Work out the finished part from the listing and answer in its coordinate system (mm). A direction names the side the tool comes from. Round coordinates to 2 decimals unless told otherwise and drop trailing zeros. Write each loop counter-clockwise with the first axis right and the second up, starting at its lowest first coordinate (ties: lowest second). Pieces come first, ordered by that corner, then holes. Notation, with made-up numbers: (46.5, 79.25) - (85.5, 79.25) arc R33 ccw to (85.5, 109.25) - close; hole circle Ø9 at (28, -22). An arc over 180 degrees is marked (long way). Answer as a JSON object with one key per item and string values.
Autodesk Inventor part; units mm, degrees
ref_plane "Work Plane1" through (0, 18.542, 0) normal (0, 1, 0) x (1, 0, 0)
ref_plane "YZ Plane" through (0, 0, 0) normal (1, 0, 0) x (0, 1, 0)
ref_plane "XZ Plane" through (0, 0, 0) normal (0, 1, 0) x (-1, 0, 0)
sketch "Sketch1" plane through (0, 0, 0) normal (0, 1, 0) x (-1, 0, 0)
  line L0 (1.27, 0) -> (11.43, 0)
  line L1 (12.7, -1.27) -> (12.7, -21.59)
  line L2 (11.43, -22.86) -> (1.27, -22.86)
  line L3 (0, -21.59) -> (0, -1.27)
  arc A0 (12.7, -1.27) -> (11.43, 0) centre (11.43, -1.27) ccw
  arc A1 (1.27, 0) -> (0, -1.27) centre (1.27, -1.27) ccw
  arc A2 (0, -21.59) -> (1.27, -22.86) centre (1.27, -21.59) ccw
  arc A3 (11.43, -22.86) -> (12.7, -21.59) centre (11.43, -21.59) ccw
  point P0 (0, 0)
  point P1 (12.7, -22.86)
  point P2 (12.7, 0)
  point P3 (0, -22.86)
  dimension "d0" = 12.7
  dimension "d1" = 22.86
  dimension "d2" = 1.27
extrude "Extrusion1" add sketch "Sketch1" along normal blind 22.86
sketch "Sketch2" plane through (0, 22.86, 0) normal (0, 1, 0) x (1, 0, 0)
  line L0 (-12.7, 21.59) -> (-12.7, 1.27)
  line L1 (-11.43, 0) -> (-1.27, 0)
  line L2 (0, 1.27) -> (0, 21.59)
  circle A0 centre (-6.35, 6.35) radius 6.35
  point P0 (0, 0)
extrude "Extrusion2" add sketch "Sketch2" along normal blind 5.08
ref_plane "Work Plane1" through (0, 18.542, 0) normal (0, 1, 0) x (1, 0, 0)
sketch "Sketch5" plane through (0, 18.542, 0) normal (0, 1, 0) x (1, 0, 0)
  line L0 (-12.7, 27.432) -> (0, 27.432)
  line L1 (-12.7, 21.59) -> (-12.7, 1.27)
  line L2 (0, 1.27) -> (0, 21.59)
  circle A0 centre (-6.35, 24.13) radius 1.016
  line L3 (0, 11.43) -> (-12.7, 11.43) construction
  line L4 (-12.7, -4.572) -> (0, -4.572)
  circle A1 centre (-6.35, -1.27) radius 1.016
  line L5 (-12.7, -4.572) -> (-12.7, 27.432)
  line L6 (0, 27.432) -> (0, -4.572)
  point P0 (0, 0)
  dimension "d13" = 16.002
  dimension "d14" = 2.032
  dimension "d15" = 25.4
extrude "Extrusion4" add sketch "Sketch5" against normal blind 2.54
sketch "Sketch6" plane through (-11.43, 0, 0) normal (0, 0, 1) x (1, 0, 0)
  line L0 (3.429, 5.334) -> (6.731, 5.334)
  line L1 (6.731, 5.334) -> (6.731, 4.318)
  line L2 (6.731, 4.318) -> (3.429, 4.318)
  line L3 (3.429, 4.318) -> (3.429, 5.334)
  line L4 (0, 0) -> (10.16, 0)
  point P0 (11.43, 0)
  point P1 (5.08, 0)
  point P2 (5.08, 4.318)
  dimension "d18" = 3.302
  dimension "d19" = 1.016
  dimension "d20" = 4.318
extrude "Extrusion5" add sketch "Sketch6" along normal blind 2.54
sketch "Sketch7" plane through (-6.35, 27.94, -6.35) normal (0, 1, 0) x (1, 0, 0)
  circle A0 centre (0, 0) radius 2.5
  point P0 (6.35, -6.35)
  dimension "d23" = 5
extrude "Extrusion6" add sketch "Sketch7" along normal blind 4.064
properties part number "Servo_With_Attachment"
Item 1: Determine the mould class of faces 1 (the cylindrical face through (-8.334, 29.944, -7.871)), 2 (the flat face through (-6, 8, 0)), 3 (the flat face through (-3.6, 27.94, -6.4)) for opening direction Y: pulls with the +Y half, pulls with the -Y half, needs draft (parallel to the pull), parting line crosses it, or undercut.
Results found:
{"face 1": "needs draft", "face 2": "undercut", "face 3": "pulls with the +Y half"}
Item 2: For faces 4 (the flat face through (-6, 8, -22.86)), 5 (the cylindrical face through (-12.338, 20.671, -22.478)), 6 (the flat face through (-6, 5.334, 1)), 7 (the flat face through (-2, 22.86, -1)), 8 (the flat face through (-11.2, 22.86, -1.5)), determine the directions among +Z, -Z, +X, -X, +Y, -Y from which every point of the face is accessible in a straight line to the end or side of a thin tool.
Results found:
{"face 4": "-Z, +X, -X, -Y", "face 5": "-Z, -X, +Y", "face 6": "+Z, +X, -X", "face 7": "+Z, +X, +Y", "face 8": "+Z, -X, +Y"}
Item 3: A cutting plane is placed at A-A (z = 1.27). Write down the section's boundary in (x, y), and give its area (3 significant figures).
Results found:
{"outline": "(-12.7, 16) - (-7.37, 16) - (-7.37, 18.54) - (-12.7, 18.54) - close; (-8, 4.32) - (-4.7, 4.32) - (-4.7, 5.33) - (-8, 5.33) - close; (-5.33, 16) - (0, 16) - (0, 18.54) - (-5.33, 18.54) - close", "area": "30.5 mm²"}
Item 4: Consider line 1 along Z through (x, y) = (-6.35, 17.2); line 2 along X through (y, z) = (17, -24); line 3 along Z through (x, y) = (-10.5, 5.5). Determine where each line is inside the solid, lowest interval first.
Results found:
{"line 1": "-27.43 to -25.15, -23.11 to 0.25, 2.29 to 4.57", "line 2": "-12.7 to -7.36, -5.34 to 0", "line 3": "-22.86 to 0"}
Item 5: A cutting plane is placed at D-D (x = -11). Write down the section's boundary in (y, z).
Results found:
{"outline": "(0, -22.86) - (16, -22.86) - (16, -27.43) - (18.54, -27.43) - (18.54, -22.86) - (22.86, -22.86) - (22.86, -10.67) - (27.94, -10.67) - (27.94, -2.03) - (22.86, -2.03) - (22.86, 0) - (18.54, 0) - (18.54, 4.57) - (16, 4.57) - (16, 0) - (0, 0) - close"}
Item 6: Each of these flat-tipped pins is pushed along its axis until it touches: P1, Ø3, axis at x = -6, y = 8, coming from the -Z side; P2, Ø3, axis at x = -3, y = 26, coming from the -Z side; P3, Ø0.8, axis at x = -6.5, z = 0.5, coming from the -Y side. Where does it stop, or does it pass through?
Results found:
{"P1": "z = -22.86", "P2": "z = -12.42", "P3": "y = 4.32"}
Item 7: A cutting plane is placed at B-B (z = -24.13). Write down the section's boundary in (x, y).
Results found:
{"outline": "(-12.7, 16) - (-7.37, 16) - (-7.37, 18.54) - (-12.7, 18.54) - close; (-5.33, 16) - (0, 16) - (0, 18.54) - (-5.33, 18.54) - close"}
Item 8: A cutting plane is placed at C-C (y = 10.5). Write down the section's boundary in (x, z), and give its area (3 significant figures).
Results found:
{"outline": "(-12.7, -21.59) arc R1.27 ccw to (-11.43, -22.86) - (-1.27, -22.86) arc R1.27 ccw to (0, -21.59) - (0, -1.27) arc R1.27 ccw to (-1.27, 0) - (-11.43, 0) arc R1.27 ccw to (-12.7, -1.27) - close", "area": "289 mm²"}
